Geometry: final body of the model. Coordinates: model frame, mm. Round coordinates to 2 decimals unless told otherwise and drop trailing zeros. Answer in a Markdown table with one row per item. Add a question column.
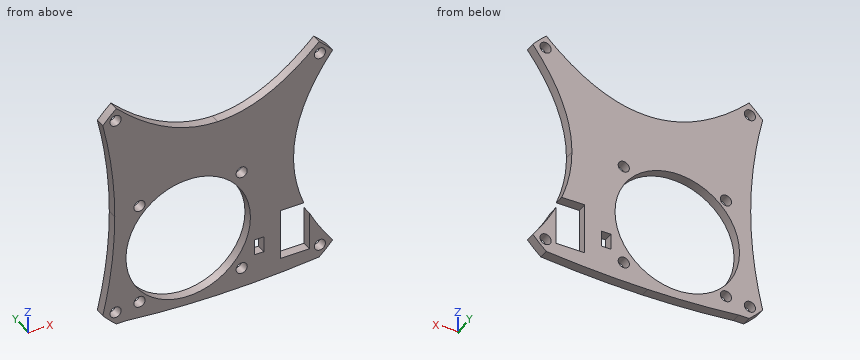
Autodesk Inventor part; units mm, degrees
ref_plane "YZ Plane" through (0, 0, 0) normal (1, 0, 0) x (0, 1, 0)
ref_plane "XZ Plane" through (0, 0, 0) normal (0, 1, 0) x (-1, 0, 0)
ref_plane "XY Plane" through (0, 0, 0) normal (0, 0, 1) x (1, 0, 0)
sketch "Sketch1" plane through (0, 0, 0) normal (0, 1, 0) x (-1, 0, 0)
  circle A0 centre (0, 0) radius 48
  dimension "d0" = 96
extrude "Extrusion1" add sketch "Sketch1" along normal blind 3
sketch "Sketch2" plane through (0, 3, 0) normal (0, 1, 0) x (1, 0, 0)
  circle A0 centre (-32, -32) radius 1.75
  line L0 (0, 0) -> (-48, 0)
  circle A1 centre (0, 0) radius 48
  line L1 (0, 0) -> (0, -48)
  circle A2 centre (32, -32) radius 1.75
  circle A3 centre (32, 32) radius 1.75
  circle A4 centre (-32, 32) radius 1.75
  dimension "d3" = 3.5
  dimension "d4" = 32
  dimension "d5" = 32
  dimension "d8" = 360
extrude "Extrusion2" cut sketch "Sketch2" against normal blind 30 contours A0 | A2 | A3 | A4
sketch "Sketch3" plane through (0, 3, 0) normal (0, 1, 0) x (1, 0, 0)
  circle A0 centre (-32, 32) radius 1.75
  line L0 (-30.25, 32) -> (-9.25, 32)
  circle A1 centre (0, 0) radius 48
  line L1 (-9.25, 32) -> (-9.25, 15.135)
  line L2 (10.25, -4.365) -> (-28.75, 34.635) construction
  line L3 (-28.75, -4.365) -> (10.25, 34.635) construction
  circle A2 centre (-9.25, 15.135) radius 19.5
  dimension "d12" = 32
  dimension "d13" = 21
  dimension "d14" = 16.865
  dimension "d17" = 39
extrude "Extrusion3" cut sketch "Sketch3" against normal blind 5 contours A2
sketch "Sketch4" plane through (0, 0, 0) normal (0, -1, 0) x (1, 0, 0)
  line L0 (-29.25, 4.865) -> (10.75, 4.865)
  line L1 (10.75, 4.865) -> (10.75, -35.135)
  line L2 (10.75, -35.135) -> (-29.25, -35.135)
  line L3 (-29.25, -35.135) -> (-29.25, 4.865)
  circle A0 centre (-9.25, -15.135) radius 19.5
  line L4 (-29.25, 4.865) -> (10.75, -35.135) construction
  line L5 (10.75, 4.865) -> (-29.25, -35.135) construction
  point P0 (0, 0)
  dimension "d20" = 40
  dimension "d21" = 40
ref_plane "Work Plane1" through (0, 3, 0) normal (0, -1, 0) x (1, 0, 0)
sketch "Sketch5" plane through (0, 3, 0) normal (0, -1, 0) x (1, 0, 0)
  circle A0 centre (7.5, -31.135) radius 1.75
  line L0 (11.5, -35.135) -> (-28.5, -35.135)
  line L1 (11.5, 4.865) -> (11.5, -35.135)
  circle A1 centre (-8.5, -15.135) radius 19.5
  circle A2 centre (-8.5, -15.135) radius 19.5
  circle A3 centre (7.5, 0.865) radius 1.75
  circle A4 centre (-24.5, 0.865) radius 1.75
  circle A5 centre (-24.5, -31.135) radius 1.75
  point P0 (0, 0)
  dimension "d24" = 3.5
  dimension "d25" = 4
  dimension "d26" = 4
  dimension "d27" = 39
  dimension "d30" = 360
extrude "Extrusion5" cut sketch "Sketch5" along normal blind 3 contours A0 | A3 | A4 | A5
sketch "Sketch7" plane through (0, 0, 0) normal (0, -1, 0) x (1, 0, 0)
  line L0 (0, 0) -> (0, 36)
  line L1 (0, 36) -> (-31.749, 36)
  circle A0 centre (0, 0) radius 48
  line L2 (0, 36) -> (31.749, 36)
  line L3 (-28.5, 4.865) -> (11.5, 4.865)
  line L4 (31.749, 36) -> (0, 4.865) construction
  line L5 (0, 4.865) -> (-31.749, 36) construction
  spline S0 degree 2 poles (31.749, 36) (0, 4.865) (-31.749, 36) knots 1 1 1 2 2 2
  dimension "d52" = 36
extrude "Extrusion7" cut sketch "Sketch7" against normal blind 5 contours S0 L1 L0 | L0 L2 S0 | L1 A0 L2
sketch "Sketch8" plane through (0, 0, 0) normal (0, -1, 0) x (1, 0, 0)
  line L0 (0, 0) -> (36, 0)
  line L1 (36, 0) -> (36, -31.749)
  arc A0 (-31.749, 36) -> (31.749, 36) centre (0, 0) ccw
  line L2 (36, 0) -> (36, 31.749)
  line L3 (11.5, 4.865) -> (11.5, -35.135)
  line L4 (36, -31.749) -> (11.5, 0) construction
  line L5 (11.5, 0) -> (36, 31.749) construction
  spline S0 degree 2 poles (36, -31.749) (11.5, 0) (36, 31.749) knots 1 1 1 2 2 2
  dimension "d55" = 36
extrude "Extrusion8" cut sketch "Sketch8" against normal blind 5
sketch "Sketch9" plane through (0, 0, 0) normal (0, -1, 0) x (1, 0, 0)
  line L0 (0, 0) -> (-36, 0)
  line L1 (-36, 0) -> (-36, 31.749)
  arc A0 (-31.749, 36) -> (36, -31.749) centre (0, 0) ccw
  line L2 (-36, 0) -> (-36, -31.749)
  line L3 (-28.5, -35.135) -> (-28.5, 4.865)
  line L4 (-36, 31.749) -> (-28.5, 0) construction
  line L5 (-28.5, 0) -> (-36, -31.749) construction
  spline S0 degree 2 poles (-36, 31.749) (-28.5, 0) (-36, -31.749) knots 1 1 1 2 2 2
  dimension "d58" = 36
extrude "Extrusion9" cut sketch "Sketch9" against normal blind 5
sketch "Sketch10" plane through (0, 0, 0) normal (0, -1, 0) x (1, 0, 0)
  line L0 (0, 0) -> (0, -36)
  line L1 (0, -36) -> (-31.749, -36)
  line L2 (0, -36) -> (31.749, -36)
  line L3 (11.5, 4.865) -> (11.5, -35.135)
  arc A0 (-36, -31.749) -> (36, -31.749) centre (0, 0) ccw
  line L4 (-28.5, -36) -> (-28.5, -38.6232)
  line L5 (-28.5, -35.135) -> (-28.5, 4.865)
  line L6 (0, -36) -> (0, -39)
  line L7 (31.749, -36) -> (0, -39) construction
  line L8 (0, -39) -> (-28.5, -36) construction
  spline S0 degree 2 poles (31.749, -36) (0, -39) (-28.5, -36) knots 1 1 1 2 2 2
  arc A1 (-31.749, -36) -> (31.749, -36) centre (0, 0) ccw
  dimension "d61" = 36
  dimension "d69" = 31.749
  dimension "d71" = 2.6232
  dimension "d72" = 3
sketch "Sketch11" plane through (0, 0, 0) normal (0, -1, 0) x (1, 0, 0)
  line L0 (11.5, 4.865) -> (11.5, -35.135)
  line L1 (11.5, -35.135) -> (11.5, -28.135)
  line L2 (11.5, -28.135) -> (14.5, -28.135)
  line L3 (14.5, -28.135) -> (14.5, -23.135)
  line L4 (14.5, -23.135) -> (11.5, -23.135)
  line L5 (11.5, -23.135) -> (11.5, -28.135)
  point P0 (0, 0)
  dimension "d64" = 7
  dimension "d65" = 3
  dimension "d66" = 5
extrude "Extrusion11" cut sketch "Sketch11" against normal blind 5
extrude "Extrusion12" cut sketch "Sketch10" against normal blind 5 contours L4 A0 L1 | S0 A0 L4
sketch "Sketch13" plane through (0, 0, 0) normal (0, -1, 0) x (1, 0, 0)
  circle A0 centre (32, -32) radius 1.75
  line L0 (32, -32) -> (28.23, -32)
  line L1 (28.23, -32) -> (28.23, -24.2)
  line L2 (28.23, -24.2) -> (24.23, -24.2)
  line L3 (19.73, -16.2) -> (28.73, -16.2)
  line L4 (28.73, -16.2) -> (28.73, -32.2)
  line L5 (28.73, -32.2) -> (19.73, -32.2)
  line L6 (19.73, -32.2) -> (19.73, -16.2)
  line L7 (19.73, -16.2) -> (28.73, -32.2) construction
  line L8 (28.73, -16.2) -> (19.73, -32.2) construction
  point P0 (0, 0)
  dimension "d82" = 3.77
  dimension "d83" = 7.8
  dimension "d84" = 4
  dimension "d85" = 9
  dimension "d86" = 16
extrude "Extrusion14" cut sketch "Sketch13" against normal blind 3 contours L3 L4 L5 L6
properties part number "Fan_Mount"
1) Contact query for flat-ended pins moving along their axis: pin 1 Ø1.5 at (y, z) = (1, -0.5) entering from +X; pin 2 Ø4.5 at (x, z) = (7.5, 0.865) entering from +Y; pin 3 Ø1.5 at (y, z) = (2, 19.5) entering from -X; pin 4 Ø1.5 at (x, y) = (-26.5, 2) entering from -Z. Output: stop coordinate, or through.
2) Material intervals for line 1 along Z through (x, y) = (-24.5, 2.3) (3 decimals); line 2 along Z through (x, y) = (32, 0.9); line 3 along Z through (x, y) = (-32, 1.7), sorted ascending. Write a range as from..to.
3) Section A-A, the plane x = 25. Give the number of separate pieces and of enclosed holes in the cut face, and give its area (3 significant figures).
Evaluation:
| question | item | result |
|---|---|---|
| 1 | pin 1 | stops at x = 23.77 |
| 1 | pin 2 | stops at y = 3 |
| 1 | pin 3 | stops at x = -33.78 |
| 1 | pin 4 | stops at z = -36.27 |
| 2 | line 1 | z = -36.39..-32.885, -29.385..-27.288, -2.982..-0.885, 2.615..29.703 |
| 2 | line 2 | z = -35.78..-33.75, -30.25..-26.05, 26.05..30.25, 33.75..35.78 |
| 2 | line 3 | z = -35.78..-33.75, -30.25..30.25, 33.75..35.78 |
| 3 | separate pieces | 3 |
| 3 | enclosed holes | 0 |
| 3 | area | 91.1 mm² |
